CAD build for the part. Positions are in the model's coordinates, mm. Face numbers are marked on the shaded views. A direction names the side the tool comes from. Coordinates: 2 decimals unless noted, no trailing zeros. Loops run counter-clockwise (first coordinate to the right, second up) from the corner with the lowest first, then second, coordinate; pieces in that order, holes last. Notation, with made-up numbers: (-13, 56.25) -> (45, 56.25) arc R28 cw to (45, 90.25) -> close; hole circle Ø6 at (71, -35). An arc over 180 degrees is marked (long way). Write each question's results on one line, items separated by ' | '.
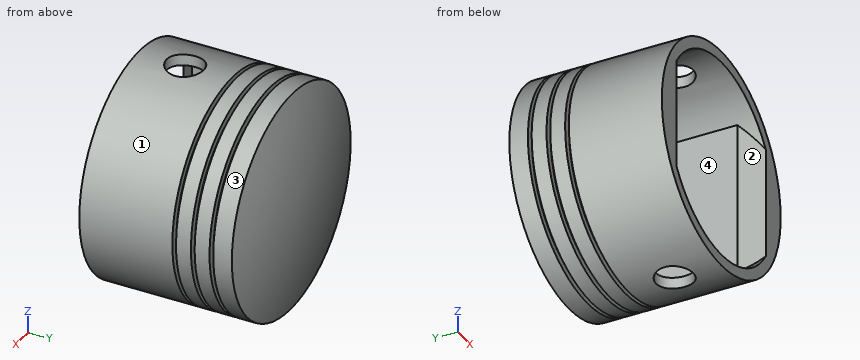
from build123d import *

# Parameters (mm, degrees)
SKETCH1_R                           = 30
BOSS_EXTRUDE1_DEPTH                 = 45
SKETCH2_W                           = 4
SKETCH2_H                           = 1
SKETCH3_R                           = 5
CUT_EXTRUDE1_DEPTH                  = 62.846584384
CUT_EXTRUDE1_DEPTH_BACK             = 62.846584384
CUT_EXTRUDE3_REACH                  = 63.847
CUT_EXTRUDE3_END_RADIUS             = 27
SKETCH8_W                           = 35
SKETCH8_H                           = 70
CUT_EXTRUDE3_DIRECTION_2_REACH      = 63.847
CUT_EXTRUDE3_DIRECTION_2_END_RADIUS = 27
SKETCH9_W                           = 15
SKETCH9_H                           = 35
SKETCH9_H_2                         = 2
CHAMFER2_SIZE                       = 5


with BuildPart() as part:
    # Sketch1 → Boss-Extrude1 (new body)
    with BuildSketch(Plane(origin=(0, 0, 0), x_dir=(1, 0, 0), z_dir=(0, 1, 0))):
        with Locations(Location((0, 0, 0), (0, 0, 90))):
            Circle(SKETCH1_R)
    extrude(amount=BOSS_EXTRUDE1_DEPTH)

    # Sketch2 → Cut-Revolve3 (revolve, cut)
    with BuildSketch(Plane.XY, mode=Mode.PRIVATE) as cut_revolve3_sk:
        with Locations((30, 25.5)):
            Rectangle(SKETCH2_W, SKETCH2_H)
        with Locations((30, 30.5)):
            Rectangle(SKETCH2_W, SKETCH2_H)
        with Locations((30, 35.5)):
            Rectangle(SKETCH2_W, SKETCH2_H)
        with BuildLine():
            Line((0, 45), (0, 47.512456789))
            Line((0, 47.512456789), (33.213865232, 47.512456789))
            Line((33.213865232, 47.512456789), (30, 41))
            ThreePointArc((30, 41), (15.13274595, 43.995594628), (0, 45))
        make_face()
    revolve(cut_revolve3_sk.sketch.rotate(Axis((0, 0, 0), (0, 1, 0)), 90), axis=Axis((0, 0, 0), (0, 1, 0)), mode=Mode.SUBTRACT)

    # Sketch3 → Cut-Extrude1 (cut, two sides)
    with BuildSketch(Plane.XY) as cut_extrude1_sk:
        with Locations((0, 12.5)):
            Circle(SKETCH3_R)
    extrude(amount=CUT_EXTRUDE1_DEPTH, mode=Mode.SUBTRACT)
    extrude(cut_extrude1_sk.sketch, amount=-CUT_EXTRUDE1_DEPTH_BACK, mode=Mode.SUBTRACT)

    # Cut-Extrude3: up to this cylinder (the profile starts inside it)
    cut_extrude3_end = Plane(origin=(0, 0, 0), z_dir=(0, -1, 0)) * Cylinder(CUT_EXTRUDE3_END_RADIUS, 182.694, mode=Mode.PRIVATE)
    # Sketch8 → Cut-Extrude3 (cut, up to the surface)
    with BuildSketch(Plane.XY, mode=Mode.PRIVATE) as cut_extrude3_sk1:
        Rectangle(SKETCH8_W, SKETCH8_H)
    cut_extrude3_tool1 = extrude(cut_extrude3_sk1.sketch, amount=-CUT_EXTRUDE3_REACH, mode=Mode.PRIVATE) & cut_extrude3_end
    add(cut_extrude3_tool1.solids().sort_by_distance((0, 0, 0))[0], mode=Mode.SUBTRACT)

    # Cut-Extrude3 direction 2: up to this cylinder (the profile starts inside it)
    cut_extrude3_direction_2_end = Plane(origin=(0, 0, 0), z_dir=(0, -1, 0)) * Cylinder(CUT_EXTRUDE3_DIRECTION_2_END_RADIUS, 182.694, mode=Mode.PRIVATE)
    # Sketch8 → Cut-Extrude3 direction 2 (cut, up to the surface)
    with BuildSketch(Plane.XY, mode=Mode.PRIVATE) as cut_extrude3_direction_2_sk1:
        Rectangle(SKETCH8_W, SKETCH8_H)
    cut_extrude3_direction_2_tool1 = extrude(cut_extrude3_direction_2_sk1.sketch, amount=CUT_EXTRUDE3_DIRECTION_2_REACH, mode=Mode.PRIVATE) & cut_extrude3_direction_2_end
    add(cut_extrude3_direction_2_tool1.solids().sort_by_distance((0, 0, 0))[0], mode=Mode.SUBTRACT)

    # Sketch9 → Cut-Revolve4 (revolve, cut)
    with BuildSketch(Plane.XY):
        with Locations((-7.5, 17.5)):
            Rectangle(SKETCH9_W, SKETCH9_H)
        with Locations((-7.5, 36)):
            Rectangle(SKETCH9_W, SKETCH9_H_2)
        Polygon((-27, 35), (-15, 35), (-15, 37), (0, 37), (0, 39), (-27, 39), align=None)
        with BuildLine():
            ThreePointArc((0, 42), (-13.583077707, 41.247699365), (-27, 39))
            Line((-27, 39), (0, 39))
            Line((0, 39), (0, 42))
        make_face()
        with BuildLine():
            Line((0, 39), (27, 39))
            ThreePointArc((27, 39), (13.583077707, 41.247699365), (0, 42))
            Line((0, 42), (0, 39))
        make_face()
    revolve(axis=Axis((0, 0, 0), (0, -1, 0)), mode=Mode.SUBTRACT)

    # Chamfer2
    chamfer2_edges = [part.edges().sort_by_distance(p)[0] for p in [
        (17.5, 0, 0),
        (-17.5, 0, 0),
    ]]
    chamfer(chamfer2_edges, length=CHAMFER2_SIZE)


solid = part.part
1) Slice it at A-A (x = 0). Count the separate pieces of the cut face and the enclosed holes in it, then the cut area to 3 significant figures.
Outcome:
separate pieces: 3 | enclosed holes: 0 | area: 334 mm^2
2) Drill centre lines: L1, parallel to X at y = 11.5, z = 0; L2, parallel to Y at x = 0, z = 28.65; L3, parallel to Z at x = 10, y = 11.5. Where is each one in solid material? Low to high. Write a range as from..to.
Outcome:
L1: x = -30..-17.5, 17.5..30 | L2: y = 0..7.5, 17.5..25, 26..30, 31..35, 36..41.36 | L3: z = -28.28..-25.08, 25.08..28.28
3) Pin check, flat tips, straight feed: pin 1 (10 mm diameter, centred on y = 23.5, z = 3.5, fed in from +X); pin 2 (7.5 mm diameter, centred on x = 21.5, z = 2, fed in from +Y); pin 3 (10 mm diameter, centred on x = 13, y = 10.5, fed in from +Z). Stop position of each tip, or through.
Outcome:
pin 1: stops at x = 30 | pin 2: stops at y = 43.6 | pin 3: stops at z = 28.91
4) Which spindle directions (+Z, -Z, +X, -X, +Y, -Y) get a long thin tool onto all of the face, cutting with end or side? Do the marked faces 1 and 2. Say none if no direction does.
Outcome:
face 1: +Y, -Y | face 2: -Y
5) Two-plate mould, pull along X, no slides. Class the marked faces 3 and 4: pulls with the +X half, pulls with the -X half, needs draft (parallel to the pull), parting line crosses it, or undercut.
Outcome:
face 3: parting line crosses it | face 4: undercut
6) Slice it at C-C (y = 37). Write the cut outline in (x, z).
Outcome:
outline: circle Ø60 at (0, 0); hole circle Ø54 at (0, 0)
